Source: three-view drawing plus pictorial views. Frame: mm from the lowest corner of the part. Give positions to 0.01 mm unless a question says otherwise; leave off trailing zeros. Loops run counter-clockwise (first coordinate to the right, second up) from the corner with the lowest first, then second, coordinate; pieces in that order, holes last.
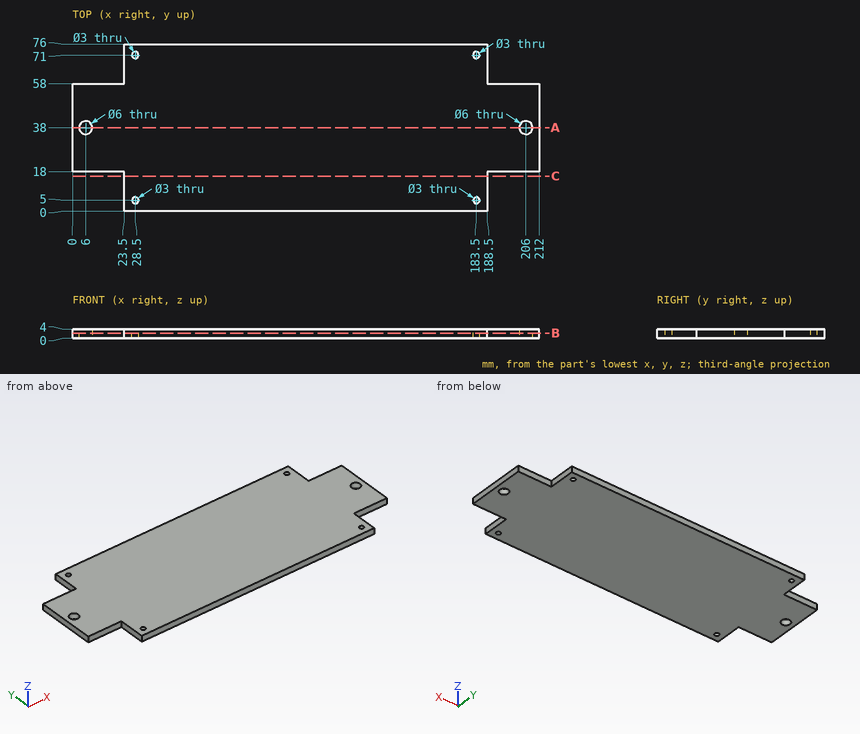
(1) Pin query (flat end, axial travel): pin 1 Ø1.2 at (y, z) = (10.5, 2.5) entering from -X; pin 2 Ø1.2 at (x, z) = (204.5, 2) entering from -Y. Return the tip coordinate at first contact, or that it passes through.
Values follow:
pin 1: stops at x = 23.5
pin 2: stops at y = 18
(2) Cut plane C-C (y = 16). Return the cut outline in (x, z), and give its area (3 significant figures).
Values follow:
outline: (23.5, 0) - (188.5, 0) - (188.5, 4) - (23.5, 4) - close
area: 660 mm2
(3) Ray query, probe 1 along Y at (x, z) = (28.5, 1.6); probe 2 along X at (y, z) = (71, 1.35); probe 3 along Y at (x, z) = (206, 2.4). Return the intervals inside material, ascending.
Values follow:
probe 1: y = 0 to 3.5, 6.5 to 69.5, 72.5 to 76
probe 2: x = 23.5 to 27, 30 to 182, 185 to 188.5
probe 3: y = 18 to 35, 41 to 58
(4) Cut plane A-A (y = 38). Return the cut outline in (x, z), and give its area (3 significant figures).
Values follow:
outline: (0, 0) - (3, 0) - (3, 4) - (0, 4) - close; (9, 0) - (203, 0) - (203, 4) - (9, 4) - close; (209, 0) - (212, 0) - (212, 4) - (209, 4) - close
area: 800 mm2
(5) Cut plane B-B (z = 2.3). Return the cut outline in (x, y), and give its area (3 significant figures).
Values follow:
outline: (0, 18) - (23.5, 18) - (23.5, 0) - (188.5, 0) - (188.5, 18) - (212, 18) - (212, 58) - (188.5, 58) - (188.5, 76) - (23.5, 76) - (23.5, 58) - (0, 58) - close; hole circle Ø6 at (6, 38); hole circle Ø3 at (28.5, 5); hole circle Ø3 at (28.5, 71); hole circle Ø3 at (183.5, 5); hole circle Ø3 at (183.5, 71); hole circle Ø6 at (206, 38)
area: 14,300 mm2
